Build history of the part. All positions in model axes, mm. Coordinates: 2 decimals unless noted, no trailing zeros.
Item 1: Cut at A-A (z = 2.95). Count the separate pieces of the cut face and the enclosed holes in it, and give its area (3 significant figures).
Item 2: Drill centre lines: line 1 along X through (y, z) = (74, 0.3); line 2 along X through (y, z) = (65, 3.05); line 3 along Y through (x, z) = (111.5, 1.6). Where is each one in solid material? Low to high.
Item 3: Flat gauge pins, fed straight in: pin 1 (12 mm diameter, centred on x = 100.5, y = -1, fed in from -Z); pin 2 (2.5 mm diameter, centred on x = 131.18, y = -65, fed in from -Z); pin 3 (2.5 mm diameter, centred on x = -85, z = 3, fed in from -Y); pin 4 (2.5 mm diameter, centred on x = -83, z = 2, fed in from +Y). Where does each tip first touch, or does it go through?
from build123d import *

# Parameters (mm, degrees)
BOSS_EXTRUDE1_OUTLINE_W   = 245.000446045
BOSS_EXTRUDE1_OUTLINE_H   = 180
BOSS_EXTRUDE1_OUTLINE_W_2 = 5
BOSS_EXTRUDE1_OUTLINE_H_2 = 5
BOSS_EXTRUDE1_OUTLINE_R   = 1.5
BOSS_EXTRUDE1_DEPTH       = 5
FILLET1_R                 = 10


# Read off the part's stored shape, not the designer's step: Boss-Extrude1
with BuildPart() as part:
    # Boss-Extrude1 outline → Boss-Extrude1 (new body)
    with BuildSketch(Plane.XY):
        with Locations((31.175821468, 0)):
            Rectangle(BOSS_EXTRUDE1_OUTLINE_W, BOSS_EXTRUDE1_OUTLINE_H)
        with Locations((-66.324847601, -82.5)):
            Rectangle(BOSS_EXTRUDE1_OUTLINE_W_2, BOSS_EXTRUDE1_OUTLINE_H_2, mode=Mode.SUBTRACT)
        with Locations((-83.824401555, -72.5)):
            Rectangle(BOSS_EXTRUDE1_OUTLINE_W_2, BOSS_EXTRUDE1_OUTLINE_H_2, mode=Mode.SUBTRACT)
        with Locations((-58.824847601, -82.5)):
            Circle(BOSS_EXTRUDE1_OUTLINE_R, mode=Mode.SUBTRACT)
        with Locations((-51.324847601, -82.5)):
            Rectangle(BOSS_EXTRUDE1_OUTLINE_W_2, BOSS_EXTRUDE1_OUTLINE_H_2, mode=Mode.SUBTRACT)
        with Locations((-83.824401555, -65)):
            Circle(BOSS_EXTRUDE1_OUTLINE_R, mode=Mode.SUBTRACT)
        with Locations((-83.824401555, -57.5)):
            Rectangle(BOSS_EXTRUDE1_OUTLINE_W_2, BOSS_EXTRUDE1_OUTLINE_H_2, mode=Mode.SUBTRACT)
        with Locations((83.67604449, -82.5)):
            Rectangle(BOSS_EXTRUDE1_OUTLINE_W_2, BOSS_EXTRUDE1_OUTLINE_H_2, mode=Mode.SUBTRACT)
        with Locations((91.17604449, -82.5)):
            Circle(BOSS_EXTRUDE1_OUTLINE_R, mode=Mode.SUBTRACT)
        with Locations((98.67604449, -82.5)):
            Rectangle(BOSS_EXTRUDE1_OUTLINE_W_2, BOSS_EXTRUDE1_OUTLINE_H_2, mode=Mode.SUBTRACT)
        with Locations((106.17604449, -82.5)):
            Circle(BOSS_EXTRUDE1_OUTLINE_R, mode=Mode.SUBTRACT)
        with Locations((113.67604449, -82.5)):
            Rectangle(BOSS_EXTRUDE1_OUTLINE_W_2, BOSS_EXTRUDE1_OUTLINE_H_2, mode=Mode.SUBTRACT)
        with Locations((121.17604449, -82.5)):
            Circle(BOSS_EXTRUDE1_OUTLINE_R, mode=Mode.SUBTRACT)
        with Locations((116.17604449, -72.5)):
            Rectangle(BOSS_EXTRUDE1_OUTLINE_W_2, BOSS_EXTRUDE1_OUTLINE_H_2, mode=Mode.SUBTRACT)
        with Locations((128.67604449, -82.5)):
            Rectangle(BOSS_EXTRUDE1_OUTLINE_W_2, BOSS_EXTRUDE1_OUTLINE_H_2, mode=Mode.SUBTRACT)
        with Locations((131.17604449, -72.5)):
            Rectangle(BOSS_EXTRUDE1_OUTLINE_W_2, BOSS_EXTRUDE1_OUTLINE_H_2, mode=Mode.SUBTRACT)
        with Locations((146.17604449, -72.5)):
            Rectangle(BOSS_EXTRUDE1_OUTLINE_W_2, BOSS_EXTRUDE1_OUTLINE_H_2, mode=Mode.SUBTRACT)
        with Locations((116.17604449, -65)):
            Circle(BOSS_EXTRUDE1_OUTLINE_R, mode=Mode.SUBTRACT)
        with Locations((116.17604449, -57.5)):
            Rectangle(BOSS_EXTRUDE1_OUTLINE_W_2, BOSS_EXTRUDE1_OUTLINE_H_2, mode=Mode.SUBTRACT)
        with Locations((131.17604449, -65)):
            Circle(BOSS_EXTRUDE1_OUTLINE_R, mode=Mode.SUBTRACT)
        with Locations((131.17604449, -57.5)):
            Rectangle(BOSS_EXTRUDE1_OUTLINE_W_2, BOSS_EXTRUDE1_OUTLINE_H_2, mode=Mode.SUBTRACT)
        with Locations((146.17604449, -65)):
            Circle(BOSS_EXTRUDE1_OUTLINE_R, mode=Mode.SUBTRACT)
        with Locations((146.17604449, -57.5)):
            Rectangle(BOSS_EXTRUDE1_OUTLINE_W_2, BOSS_EXTRUDE1_OUTLINE_H_2, mode=Mode.SUBTRACT)
        with Locations((-83.824401555, 57.5)):
            Rectangle(BOSS_EXTRUDE1_OUTLINE_W_2, BOSS_EXTRUDE1_OUTLINE_H_2, mode=Mode.SUBTRACT)
        with Locations((-83.824401555, 65)):
            Circle(BOSS_EXTRUDE1_OUTLINE_R, mode=Mode.SUBTRACT)
        with Locations((-83.824401555, 72.5)):
            Rectangle(BOSS_EXTRUDE1_OUTLINE_W_2, BOSS_EXTRUDE1_OUTLINE_H_2, mode=Mode.SUBTRACT)
        with Locations((-66.324847601, 82.5)):
            Rectangle(BOSS_EXTRUDE1_OUTLINE_W_2, BOSS_EXTRUDE1_OUTLINE_H_2, mode=Mode.SUBTRACT)
        with Locations((-58.824847601, 82.5)):
            Circle(BOSS_EXTRUDE1_OUTLINE_R, mode=Mode.SUBTRACT)
        with Locations((-51.324847601, 82.5)):
            Rectangle(BOSS_EXTRUDE1_OUTLINE_W_2, BOSS_EXTRUDE1_OUTLINE_H_2, mode=Mode.SUBTRACT)
        with Locations((83.676044481, 82.5)):
            Rectangle(BOSS_EXTRUDE1_OUTLINE_W_2, BOSS_EXTRUDE1_OUTLINE_H_2, mode=Mode.SUBTRACT)
        with Locations((91.176044481, 82.5)):
            Circle(BOSS_EXTRUDE1_OUTLINE_R, mode=Mode.SUBTRACT)
        with Locations((116.17604449, 57.5)):
            Rectangle(BOSS_EXTRUDE1_OUTLINE_W_2, BOSS_EXTRUDE1_OUTLINE_H_2, mode=Mode.SUBTRACT)
        with Locations((116.17604449, 65)):
            Circle(BOSS_EXTRUDE1_OUTLINE_R, mode=Mode.SUBTRACT)
        with Locations((131.17604449, 57.5)):
            Rectangle(BOSS_EXTRUDE1_OUTLINE_W_2, BOSS_EXTRUDE1_OUTLINE_H_2, mode=Mode.SUBTRACT)
        with Locations((131.17604449, 65)):
            Circle(BOSS_EXTRUDE1_OUTLINE_R, mode=Mode.SUBTRACT)
        with Locations((146.17604449, 57.5)):
            Rectangle(BOSS_EXTRUDE1_OUTLINE_W_2, BOSS_EXTRUDE1_OUTLINE_H_2, mode=Mode.SUBTRACT)
        with Locations((146.17604449, 65)):
            Circle(BOSS_EXTRUDE1_OUTLINE_R, mode=Mode.SUBTRACT)
        with Locations((116.17604449, 72.5)):
            Rectangle(BOSS_EXTRUDE1_OUTLINE_W_2, BOSS_EXTRUDE1_OUTLINE_H_2, mode=Mode.SUBTRACT)
        with Locations((98.67604449, 82.5)):
            Rectangle(BOSS_EXTRUDE1_OUTLINE_W_2, BOSS_EXTRUDE1_OUTLINE_H_2, mode=Mode.SUBTRACT)
        with Locations((106.17604449, 82.5)):
            Circle(BOSS_EXTRUDE1_OUTLINE_R, mode=Mode.SUBTRACT)
        with Locations((113.67604449, 82.5)):
            Rectangle(BOSS_EXTRUDE1_OUTLINE_W_2, BOSS_EXTRUDE1_OUTLINE_H_2, mode=Mode.SUBTRACT)
        with Locations((121.17604449, 82.5)):
            Circle(BOSS_EXTRUDE1_OUTLINE_R, mode=Mode.SUBTRACT)
        with Locations((131.17604449, 72.5)):
            Rectangle(BOSS_EXTRUDE1_OUTLINE_W_2, BOSS_EXTRUDE1_OUTLINE_H_2, mode=Mode.SUBTRACT)
        with Locations((146.17604449, 72.5)):
            Rectangle(BOSS_EXTRUDE1_OUTLINE_W_2, BOSS_EXTRUDE1_OUTLINE_H_2, mode=Mode.SUBTRACT)
        with Locations((128.67604449, 82.5)):
            Rectangle(BOSS_EXTRUDE1_OUTLINE_W_2, BOSS_EXTRUDE1_OUTLINE_H_2, mode=Mode.SUBTRACT)
    extrude(amount=BOSS_EXTRUDE1_DEPTH)

    # Fillet1
    fillet1_edges = [part.edges().sort_by_distance(p)[0] for p in [
        (153.67604449, -90, 2.5),
        (-91.324401555, -90, 2.5),
        (-91.324401555, 90, 2.5),
        (153.67604449, 90, 2.5),
    ]]
    fillet(fillet1_edges, radius=FILLET1_R)


solid = part.part
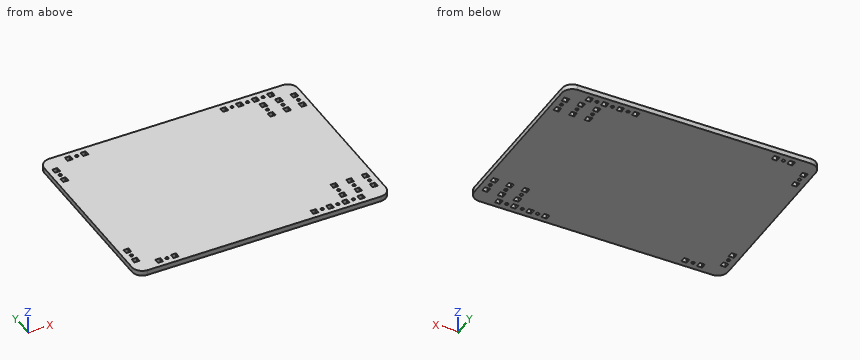
Filled sheet:
1. separate pieces: 1
1. enclosed holes: 44
1. area: 43,200 mm2
2. line 1: x = -91.32 to -86.32, -81.32 to 113.68, 118.68 to 128.68, 133.68 to 143.68, 148.68 to 153.68
2. line 2: x = -91.32 to -85.32, -82.32 to 114.68, 117.68 to 129.68, 132.68 to 144.68, 147.68 to 153.68
2. line 3: y = -90 to -85, -80 to 80, 85 to 90
3. pin 1: stops at z = 0
3. pin 2: passes through
3. pin 3: stops at y = -89.7
3. pin 4: stops at y = 89.99
